Work out the finished part from the listing and answer in its coordinate system (mm). A direction names the side the tool comes from. Give positions to 0.01 mm unless a question says otherwise; leave off trailing zeros. Loops run counter-clockwise (first coordinate to the right, second up) from the corner with the lowest first, then second, coordinate; pieces in that order, holes last. Notation, with made-up numbers: (-6.75, 45) -> (24.25, 45) arc R19 ccw to (24.25, 49) -> close; hole circle Ø3 at (80.5, 37). An arc over 180 degrees is marked (long way). Answer as CSV lines item,"result". Start each with the question number.
1. Find the intervals of material crossed by line 1 along X through (y, z) = (0.95, 4); line 2 along Y through (x, z) = (60.44, 5.7) (3 decimals); line 3 along Y through (x, z) = (60.44, 1.65) (3 decimals), in increasing order.
2. Find section A-A, the plane y = 12. Give the vertices of the cut face in (x, z).
3. A tool of negligible diameter and unlimited length cuts with its end or side. For faces 4 (the face through (60, 6, 3)), 5 (the face through (-3.476, 1.479, -0.783)), 6 (the face through (4.138, 1.528, -0.618)), 7 (the face through (4.99, 5.82, -1.52)), from which of +Z, -Z, +X, -X, +Y, -Y can it reach the whole face along a straight path? Write none if from no direction.
4. Find section C-C, the plane x = 46. Give the vertices of the cut face in (y, z), and give its area (3 significant figures).
5. Determine the mould class of faces 1 (the face through (4.099, 25.938, -0.042)), 2 (the face through (-0.3, 1.52, -3.19)), 3 (the face through (6.44, 5.87, 5.96)) for opening direction Y: +Y half, -Y half, draft (parallel to the pull), parting line (faces both ways), or undercut.
6. Find section B-B, the plane x = 4.56. Give the vertices of the cut face in (y, z) (3 decimals).
7. Flat-ended cylindrical pins translate along their axes: pin 1 Ø2 at (y, z) = (14.5, 1.5) entering from -X; pin 2 Ø9 at (x, y) = (28.5, 13) entering from +Z; pin 3 Ø3 at (x, y) = (60, 27.5) entering from -Z; pin 4 Ø1.2 at (x, y) = (4.56, 7.775) entering from +Z. Find the tip coordinate at first contact, or state that the pin passes through.
from build123d import *

# Parameters (mm, degrees)
SKETCH2_W           = 65
SKETCH2_H           = 30.000000000000004
BOSS_EXTRUDE1_DEPTH = 3
SKETCH3_R           = 0.9999999999999981
SKETCH3_R_2         = 0.9999999999999983
SKETCH3_R_3         = 1.0000000000000002
BOSS_EXTRUDE2_DEPTH = 3
FILLET1_R           = 10
FILLET2_R           = 1
FILLET3_R           = 1
FILLET4_R           = 5
SKETCH4_R           = 1.0000000000000004
SKETCH4_R_2         = 0.9999999999999983
CUT_EXTRUDE1_DEPTH  = 10
BOSS_EXTRUDE3_START = 3
SKETCH5_R           = 2.000000000000001
SKETCH5_R_2         = 1.0000000000000004
SKETCH5_R_3         = 2.0000000000000004
SKETCH5_R_4         = 1.0000000000000009
SKETCH5_R_5         = 2.0000000000000036
SKETCH5_R_6         = 1.000000000000005
SKETCH5_R_7         = 2.0000000000000027
SKETCH5_R_8         = 0.9999999999999983
BOSS_EXTRUDE3_DEPTH = 3
SKETCH6_R           = 2.0000000000000036
SKETCH6_R_2         = 0.9999999999999983
SKETCH6_R_3         = 2.000000000000003
SKETCH6_R_4         = 0.9999999999999981
SKETCH6_R_5         = 2
SKETCH6_R_6         = 1.0000000000000018
SKETCH6_R_7         = 1.9999999999999987
SKETCH6_R_8         = 1.0000000000000007
BOSS_EXTRUDE4_DEPTH = 6


with BuildPart() as part:
    # Sketch2 → Boss-Extrude1 (new body)
    with BuildSketch(Plane.XY):
        with Locations((32.5, 15.000000000000002)):
            Rectangle(SKETCH2_W, SKETCH2_H)
    extrude(amount=BOSS_EXTRUDE1_DEPTH)

    # Sketch3 → Boss-Extrude2 (add)
    # profile 1 of 2: a face of its own
    with BuildSketch(Plane.XZ):
        Polygon((65, 1.5), (65, 6.500000000000001), (70, 6.500000000000001), (70, -3.4999999999999996), (65, -3.4999999999999996), align=None)
        with Locations(Location((67.5, 4, 0), (0, 0, 270))):
            Circle(SKETCH3_R, mode=Mode.SUBTRACT)
        with Locations(Location((67.5, -1, 0), (0, 0, 270))):
            Circle(SKETCH3_R_2, mode=Mode.SUBTRACT)
    # profile 2 of 2: a face of its own
    with BuildSketch(Plane.XZ):
        Polygon((-5, 1.4999999999999993), (-5, 6.5), (0, 6.5), (0, -3.5000000000000013), (-5, -3.5000000000000018), align=None)
        with Locations(Location((-2.5, 3.999999999999999, 0), (0, 0, 270))):
            Circle(SKETCH3_R_3, mode=Mode.SUBTRACT)
        with Locations(Location((-2.5, -1.0000000000000018, 0), (0, 0, 270))):
            Circle(SKETCH3_R_3, mode=Mode.SUBTRACT)
    extrude(amount=-BOSS_EXTRUDE2_DEPTH)

    # Fillet1
    # the kernel refuses this fillet: 10 mm, written as the material it adds along each edge
    with BuildSketch(Plane(origin=(65, 3, 3), x_dir=(-1, 0, 0), z_dir=(0, -1, 0))) as fillet1_piece_1:
        with BuildLine():
            CenterArc((7.599342076785334, -10), FILLET1_R, 90, 49.458398126495496)
            Line((0, -3.500000000000001), (0, 0))
            Line((0, 0), (7.599342076785334, 0))
        make_face()
    extrude(amount=3)
    with BuildSketch(Plane(origin=(65, 3, 0), x_dir=(-1, 0, 0), z_dir=(0, -1, 0))) as fillet1_piece_2:
        with BuildLine():
            CenterArc((7.599342076785334, 10), FILLET1_R, 220.5416018735045, 49.45839812649547)
            Line((0, 3.500000000000001), (0, 0))
            Line((0, 0), (7.599342076785334, 0))
        make_face()
    extrude(amount=3)
    with BuildSketch(Plane(origin=(0, 0, 0), x_dir=(1, 0, 0), z_dir=(0, 1, 0))) as fillet1_piece_3:
        with BuildLine():
            CenterArc((7.599342076785334, 10), FILLET1_R, 220.5416018735045, 49.45839812649547)
            Line((0, 3.5000000000000018), (0, 0))
            Line((0, 0), (7.599342076785334, 0))
        make_face()
    extrude(amount=3)
    with BuildSketch(Plane(origin=(0, 0, 3), x_dir=(1, 0, 0), z_dir=(0, 1, 0))) as fillet1_piece_4:
        with BuildLine():
            CenterArc((7.59934207678533, -10), FILLET1_R, 90, 49.45839812649547)
            Line((-1.78e-15, -3.4999999999999982), (0, 0))
            Line((0, 0), (7.59934207678533, 0))
        make_face()
    extrude(amount=3)

    # Fillet2
    fillet2_edges = [part.edges().sort_by_distance(p)[0] for p in [
        (70, 1.5, 6.500000000000001),
        (70, 1.5, -3.4999999999999996),
        (-5, 1.5, -3.5000000000000018),
        (-5, 1.5, 6.5),
    ]]
    fillet(fillet2_edges, radius=FILLET2_R)

    # Fillet3
    fillet3_edges = [part.edges().sort_by_distance(p)[0] for p in [
        (0, 3, 1.5),
        (65, 16.5, 0),
        (65, 16.5, 3),
        (65, 3, 1.5),
        (0, 16.5, 3),
        (0, 16.5, 0),
        (3.7996710383925, 3, 3),
        (61.2003289616075, 3, 3),
        (3.7996710383925, 3, 0),
        (61.2003289616075, 3, 0),
    ]]
    fillet(fillet3_edges, radius=FILLET3_R)

    # Fillet4
    fillet4_edges = [part.edges().sort_by_distance(p)[0] for p in [
        (65, 1.5, -3.4999999999999996),
        (65, 1.5, 6.500000000000001),
        (0, 1.5, 6.5),
        (0, 1.5, -3.5000000000000013),
    ]]
    fillet(fillet4_edges, radius=FILLET4_R)

    # Sketch4 → Cut-Extrude1 (cut)
    with BuildSketch(Plane(origin=(0, 0, 0), x_dir=(-1, 0, 0), z_dir=(0, 0, -1))):
        with Locations((-4.559999999999932, 26.825000000000006)):
            Circle(SKETCH4_R)
        with Locations((-60.439999999999934, 26.825000000000006)):
            Circle(SKETCH4_R_2)
        with Locations((-60.439999999999934, 7.775000000000004)):
            Circle(SKETCH4_R_2)
        with Locations((-4.559999999999932, 7.775000000000004)):
            Circle(SKETCH4_R)
    extrude(amount=-CUT_EXTRUDE1_DEPTH, mode=Mode.SUBTRACT)

    # Sketch5 → Boss-Extrude3 (add)
    # profile 1 of 4: a face of its own
    with BuildSketch(Plane(origin=(0, 0, 0), x_dir=(-1, 0, 0), z_dir=(0, 0, -1)).offset(BOSS_EXTRUDE3_START)):
        with Locations((-4.559999999999932, 26.825000000000006)):
            Circle(SKETCH5_R)
        with Locations((-4.559999999999932, 26.825000000000006)):
            Circle(SKETCH5_R_2, mode=Mode.SUBTRACT)
    # profile 2 of 4: a face of its own
    with BuildSketch(Plane(origin=(0, 0, 0), x_dir=(-1, 0, 0), z_dir=(0, 0, -1)).offset(BOSS_EXTRUDE3_START)):
        with Locations((-4.559999999999932, 7.775000000000004)):
            Circle(SKETCH5_R_3)
        with Locations((-4.559999999999932, 7.775000000000004)):
            Circle(SKETCH5_R_4, mode=Mode.SUBTRACT)
    # profile 3 of 4: a face of its own
    with BuildSketch(Plane(origin=(0, 0, 0), x_dir=(-1, 0, 0), z_dir=(0, 0, -1)).offset(BOSS_EXTRUDE3_START)):
        with Locations((-60.439999999999934, 26.825000000000006)):
            Circle(SKETCH5_R_5)
        with Locations((-60.439999999999934, 26.825000000000006)):
            Circle(SKETCH5_R_6, mode=Mode.SUBTRACT)
    # profile 4 of 4: a face of its own
    with BuildSketch(Plane(origin=(0, 0, 0), x_dir=(-1, 0, 0), z_dir=(0, 0, -1)).offset(BOSS_EXTRUDE3_START)):
        with Locations((-60.439999999999934, 7.775000000000004)):
            Circle(SKETCH5_R_7)
        with Locations((-60.439999999999934, 7.775000000000004)):
            Circle(SKETCH5_R_8, mode=Mode.SUBTRACT)
    extrude(amount=-BOSS_EXTRUDE3_DEPTH)

    # Sketch6 → Boss-Extrude4 (add)
    # profile 1 of 4: a face of its own
    with BuildSketch(Plane.XY.offset(3)):
        with Locations(Location((60.439999999999934, 26.825000000000006, 0), (0, 0, 180))):
            Circle(SKETCH6_R)
        with Locations(Location((60.439999999999934, 26.825000000000006, 0), (0, 0, 180))):
            Circle(SKETCH6_R_2, mode=Mode.SUBTRACT)
    # profile 2 of 4: a face of its own
    with BuildSketch(Plane.XY.offset(3)):
        with Locations(Location((60.439999999999934, 5.825000000000004, 0), (0, 0, 119.294600838))):
            Circle(SKETCH6_R_3)
        with Locations(Location((60.439999999999934, 5.825000000000004, 0), (0, 0, 102.838568141))):
            Circle(SKETCH6_R_4, mode=Mode.SUBTRACT)
    # profile 3 of 4: a face of its own
    with BuildSketch(Plane.XY.offset(3)):
        with Locations(Location((7.439999999999933, 26.825, 0), (0, 0, 191.357748332))):
            Circle(SKETCH6_R_5)
        with Locations((7.439999999999933, 26.825)):
            Circle(SKETCH6_R_6, mode=Mode.SUBTRACT)
    # profile 4 of 4: a face of its own
    with BuildSketch(Plane.XY.offset(3)):
        with Locations(Location((7.4399999999999356, 5.824999999999997, 0), (0, 0, 245.853152003))):
            Circle(SKETCH6_R_7)
        with Locations((7.4399999999999356, 5.824999999999997)):
            Circle(SKETCH6_R_8, mode=Mode.SUBTRACT)
    extrude(amount=BOSS_EXTRUDE4_DEPTH)


solid = part.part
Resolved:
1,line 1,"x = -5 to -3.5, -1.5 to 3.24, 61.76 to 66.5, 68.5 to 70"
1,line 2,"y = 3.825 to 4.825, 6.825 to 7.825, 24.825 to 25.825, 27.825 to 28.825"
1,line 3,"y = 0 to 6.775, 8.775 to 25.825, 27.825 to 30"
2,outline,"(0, 1) arc R1 ccw to (1, 0) -> (64, 0) arc R1 ccw to (65, 1) -> (65, 2) arc R1 ccw to (64, 3) -> (1, 3) arc R1 ccw to (0, 2) -> close"
3,face 4,"+Z"
3,face 5,"+Y, -Y"
3,face 6,"-Z, -Y"
3,face 7,"-Z"
4,outline,"(0, 0) -> (30, 0) -> (30, 3) -> (0, 3) -> close"
4,area,"90.0 mm^2"
5,face 1,"undercut"
5,face 2,"draft"
5,face 3,"undercut"
6,outline,"(0, -0.473) -> (3.15, -0.473) arc R1 cw to (4, 0) -> (5.775, 0) -> (5.775, -3) -> (6.775, -3) -> (6.775, 3) -> (4, 3) arc R1 cw to (3.15, 3.473) -> (0, 3.473) -> close; (8.775, -3) -> (9.775, -3) -> (9.775, 0) -> (24.825, 0) -> (24.825, -3) -> (25.825, -3) -> (25.825, 3) -> (8.775, 3) -> close; (27.825, -3) -> (28.825, -3) -> (28.825, 0) -> (30, 0) -> (30, 3) -> (27.825, 3) -> close"
7,pin 1,"stops at x = 0"
7,pin 2,"stops at z = 3"
7,pin 3,"stops at z = -3"
7,pin 4,"passes through"
